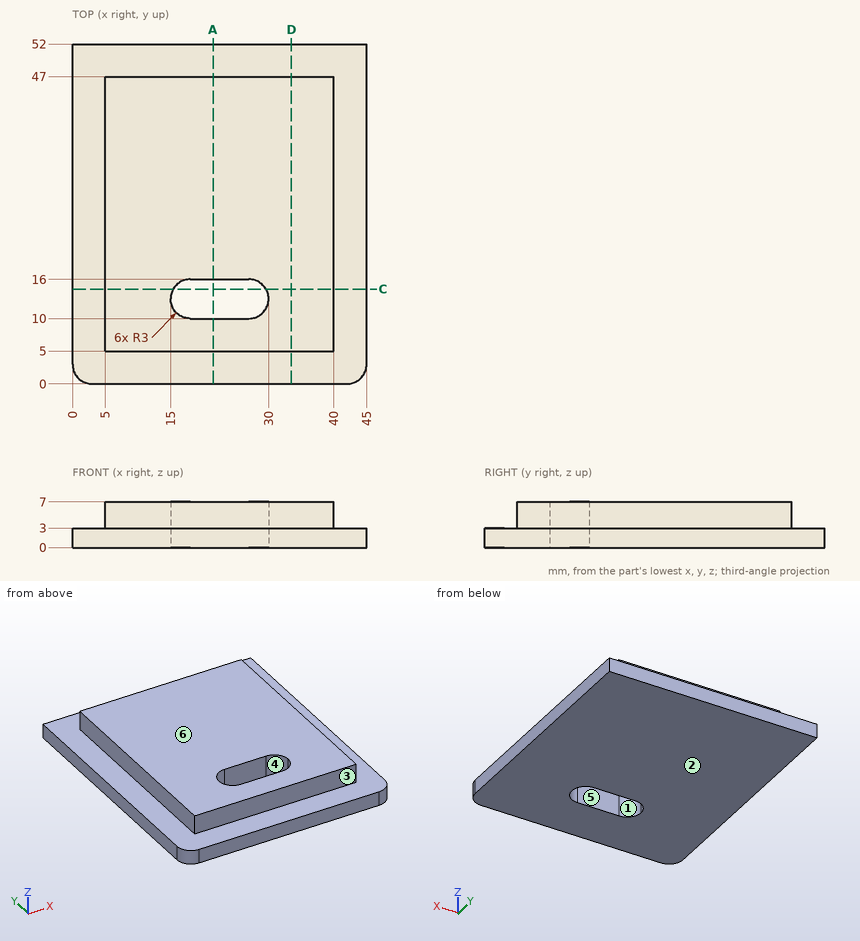
Study the drawing (mm; zero at the part's minimum x, y, z) and answer. A direction names the side the tool comes from. Coordinates: 2 decimals unless noted, no trailing zeros. Loops run counter-clockwise (first coordinate to the right, second up) from the corner with the lowest first, then second, coordinate; pieces in that order, holes last. Notation, with made-up numbers: (9, 24.25) -> (33, 24.25) arc R23 cw to (33, 53.25) -> close; hole circle Ø2 at (39.25, 27). An arc over 180 degrees is marked (long way). Answer in a Markdown table with one row per item. Add a question column.
1. Determine the mould class of the marked faces 3, 4, 5 and 6 for opening direction Y: +Y half, -Y half, draft (parallel to the pull), parting line (faces both ways), or undercut.
2. The part is cut by section D-D, the plane x = 33.5. Write down the section's boundary in (y, z), then the cut area to 3 significant figures.
3. Flat-ended cylindrical pins translate along their axes: P1, Ø1.2, axis at y = 34, z = 5.5, coming from the +X side; P2, Ø3.5, axis at x = 22, z = 5, coming from the +Y side. Find the tip coordinate at first contact, or state that the pin passes through.
4. Consider line 1 (Y direction, x = 19, z = 0.75); line 2 (Y direction, x = 26, z = 6); line 3 (X direction, y = 24, z = 5). Determine where each line is inside the solid, lowest interval first. Write a range as [from, to].
5. For the marked faces 1 and 2, determine the directions among +Z, -Z, +X, -X, +Y, -Y from which every point of the face is accessible in a straight line to the end or side of a thin tool.
6. The part is cut by section C-C, the plane y = 14.5. Write down the section's boundary in (x, z), then the cut area to 3 significant figures.
7. The part is cut by section A-A, the plane x = 21.5. Write down the section's boundary in (y, z), then the cut area to 3 significant figures.
Answer below:
| question | item | result |
|---|---|---|
| 1 | face 3 | -Y half |
| 1 | face 4 | undercut |
| 1 | face 5 | undercut |
| 1 | face 6 | draft |
| 2 | outline | (0, 0) -> (52, 0) -> (52, 3) -> (47, 3) -> (47, 7) -> (5, 7) -> (5, 3) -> (0, 3) -> close |
| 2 | area | 324 mm2 |
| 3 | P1 | x = 40 |
| 3 | P2 | y = 47 |
| 4 | line 1 | [0, 10], [16, 52] |
| 4 | line 2 | [5, 10], [16, 47] |
| 4 | line 3 | [5, 40] |
| 5 | face 1 | +Z, -Z |
| 5 | face 2 | -Z, +X, -X, +Y, -Y |
| 6 | outline | (0, 0) -> (15.4, 0) -> (15.4, 7) -> (5, 7) -> (5, 3) -> (0, 3) -> close; (29.6, 0) -> (45, 0) -> (45, 3) -> (40, 3) -> (40, 7) -> (29.6, 7) -> close |
| 6 | area | 176 mm2 |
| 7 | outline | (0, 0) -> (10, 0) -> (10, 7) -> (5, 7) -> (5, 3) -> (0, 3) -> close; (16, 0) -> (52, 0) -> (52, 3) -> (47, 3) -> (47, 7) -> (16, 7) -> close |
| 7 | area | 282 mm2 |
